Part model, mm, in its own coordinate system. Give positions to 0.01 mm unless a question says otherwise; leave off trailing zeros. Order: outer loops, then holes, each group sorted by start corner. A loop starts at its lowest first (then second) coordinate and runs counter-clockwise, first axis right, second up.
1. Slice it at A-A on y = 4.5. List the corners of the cut face in (x, z).
2. Drop flat-ended pins along their axis: pin 1 Ø10 at (x, y) = (33.5, 4.5) entering from +Z; pin 2 Ø16 at (x, z) = (34.22, 20.23) entering from +Y; pin 3 Ø8 at (y, z) = (11.5, 33.5) entering from -X; pin 4 Ø12 at (x, z) = (34.22, 20.23) entering from -Y. Give the stop position or say it passes through.
3. Probe line 1 (X direction, y = 24.5, z = 23.5); line 2 (X direction, y = 13.75, z = 21); line 3 (Z direction, x = 26.5, y = 14.5). List the from-to ranges inside material, lowest first.
Solid Edge part; units mm, degrees
sketch "Sketch1" plane through (0, 0, 0) normal (0, -1, 0) x (1, 0, 0)
  circle A0 centre (34.2218, 20.2251) radius 7.5
  circle A1 centre (34.2218, 20.2251) radius 15
extrude "Protrusion1" add sketch "Sketch1" against normal blind 30
sketch "Sketch2" plane through (34.2218, 30, 20.2251) normal (0, 1, 0) x (1, 0, 0)
  circle A0 centre (0, 0) radius 17.5
extrude "ExtrudedProtrusion_2" add sketch "Sketch2" against normal blind 30
sketch "Sketch3" plane through (34.2218, 30, 20.2251) normal (0, 1, 0) x (1, 0, 0)
  circle A0 centre (0, 0) radius 7.5
extrude "ExtrudedCutout_1" cut sketch "Sketch3" against normal blind 30
draft "Draft_1" angle 9.46 neutral plane through (34.2218, 30, 20.2251) normal (0, 1, 0) pull direction (0, 1, 0) face at (43.9062, 5.3, 5.649) face at (38.3722, 5.3, 13.9782)
sketch "Sketch4" plane through (34.2218, 30, 20.2251) normal (0, 1, 0) x (1, 0, 0)
  circle A0 centre (0, 0) radius 7.5
extrude "ExtrudedCutout_2" cut sketch "Sketch4" against normal blind 30
sketch "Sketch5" plane through (34.2218, 30, 20.2251) normal (0, 1, 0) x (1, 0, 0)
  circle A0 centre (0, 0) radius 10
extrude "ExtrudedCutout_3" cut sketch "Sketch5" against normal blind 2
sketch "Sketch6" plane through (34.2218, 0, 20.2251) normal (0, -1, 0) x (-1, 0, 0)
  circle A0 centre (0, 0) radius 10
extrude "ExtrudedCutout_4" cut sketch "Sketch6" against normal blind 2
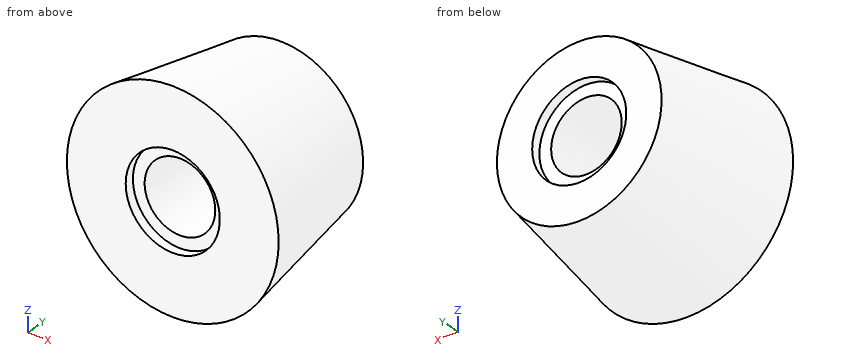
Data:
1. outline: circle Ø43.5 at (34.22, 20.23); hole circle Ø15 at (34.22, 20.23)
2. pin 1: stops at z = 42.72
2. pin 2: stops at y = 28
2. pin 3: stops at x = 15.71
2. pin 4: passes through
3. line 1: x = 16.1 to 27.47, 40.97 to 52.34
3. line 2: x = 14.03 to 26.76, 41.68 to 54.41
3. line 3: z = 1.69 to 38.76
